Job drawing, mm, ordinate dimensions from the low corner. One solid piece. Give positions to 0.01 mm unless a question says otherwise; leave off trailing zeros. Write each loop counter-clockwise with the first axis right and the second up, starting at its lowest first coordinate (ties: lowest second). Pieces come first, ordered by that corner, then holes. Notation, with made-up numbers: (-32.5, 8.25) -> (-26.5, 8.25) arc R5 cw to (-26.5, 15.25) -> close; hole circle Ø11 at (68.25, -18). An arc over 180 degrees is marked (long way). One line per question, with ' | ' between items. Start each with the question number.
(1) Drill centre lines: probe 1 along X at (y, z) = (54.5, 9.5); probe 2 along Z at (x, y) = (10.5, 8.5); probe 3 along Y at (x, z) = (47, 6.5). Where is each one in solid material? Low to high. Write a range as from..to.
(2) Band-saw the part on C-C, the plane x = 9. Give the cut face in (y, z).
(3) Pin check, flat tips, straight feed: P1, Ø1, axis at x = 36, z = 10.5, coming from the +Y side; P2, Ø1.8, axis at x = 23, z = 9, coming from the -Y side. Stop position of each tip, or through.
(4) Band-saw the part on B-B, the plane y = 100.5. Give the cut face in (x, z).
(5) Pull direction X, two halves, no side cores. Call the marked faces 1, 2 and 3: released by +X, released by -X, zero draft, split by the parting line, or undercut.
(6) Band-saw the part on A-A, the plane z = 10. Give the cut face in (x, y), and give its area (3 significant figures).
(7) Band-saw the part on D-D, the plane y = 130.5. Give the cut face in (x, z).
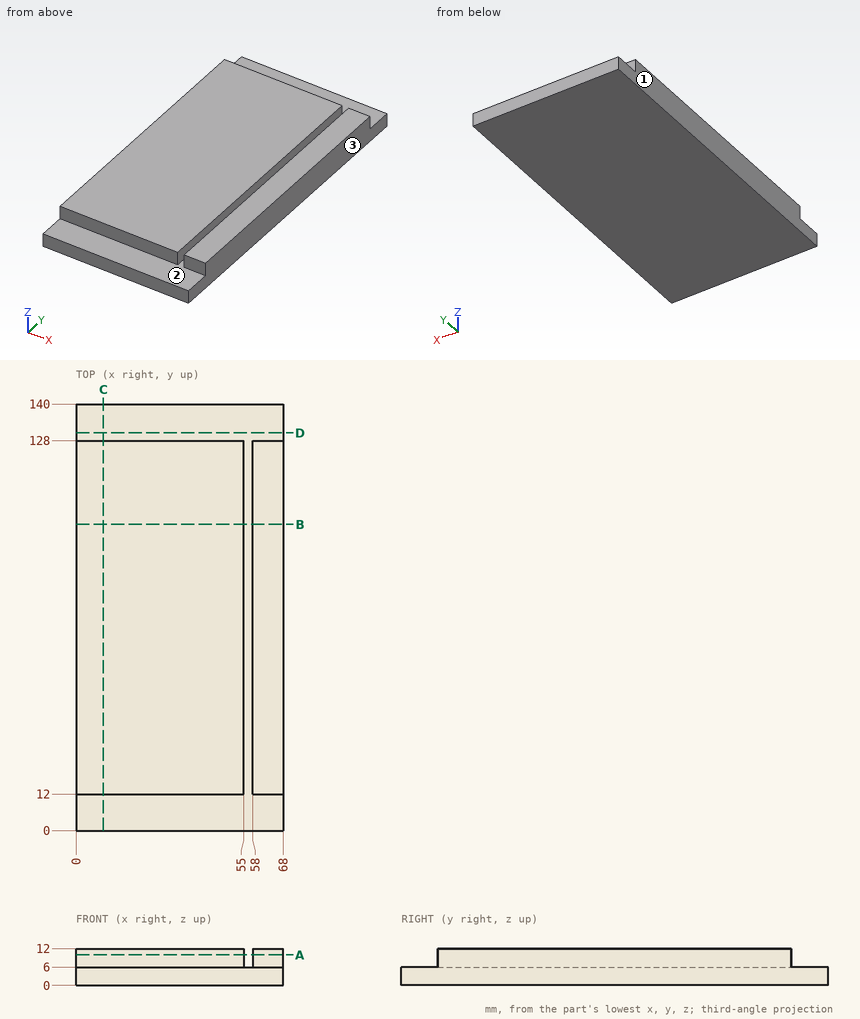
Results:
1) probe 1: x = 0..55, 58..68 | probe 2: z = 0..6 | probe 3: y = 12..128
2) outline: (0, 0) -> (140, 0) -> (140, 6) -> (128, 6) -> (128, 12) -> (12, 12) -> (12, 6) -> (0, 6) -> close
3) P1: stops at y = 128 | P2: stops at y = 12
4) outline: (0, 0) -> (68, 0) -> (68, 12) -> (58, 12) -> (58, 6) -> (55, 6) -> (55, 12) -> (0, 12) -> close
5) face 1: released by -X | face 2: undercut | face 3: released by +X
6) outline: (0, 12) -> (55, 12) -> (55, 128) -> (0, 128) -> close; (58, 12) -> (68, 12) -> (68, 128) -> (58, 128) -> close | area: 7,540 mm²
7) outline: (0, 0) -> (68, 0) -> (68, 6) -> (0, 6) -> close
